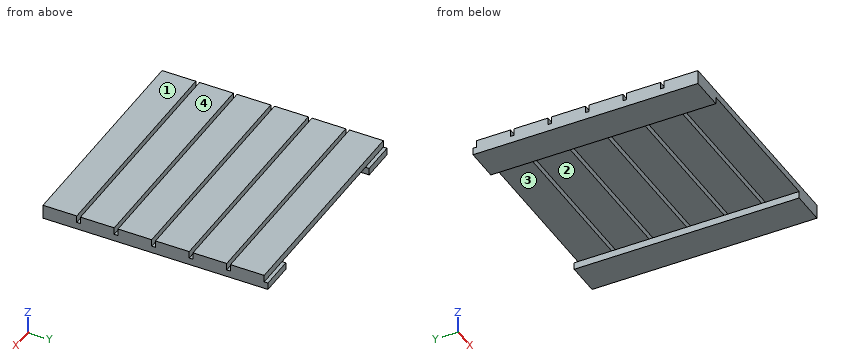
from build123d import *

# Parameters (mm, degrees)
BOX077_W     = 600
BOX077_H     = 90
BOX077_DEPTH = 19
BOX076_W     = 600
BOX076_H     = 90
BOX076_DEPTH = 19
BOX082_W     = 90
BOX082_H     = 600
BOX082_DEPTH = 19
BOX079_W     = 600
BOX079_H     = 90
BOX079_DEPTH = 19
BOX078_W     = 600
BOX078_H     = 90
BOX078_DEPTH = 19
BOX081_W     = 600
BOX081_H     = 90
BOX081_DEPTH = 19
BOX080_W     = 600
BOX080_H     = 90
BOX080_DEPTH = 19
BOX083_W     = 90
BOX083_H     = 600
BOX083_DEPTH = 19


with BuildPart() as cube049:
    # Box077 → Box077 (new body)
    with BuildSketch(Plane(origin=(0, 100, 0), x_dir=(1, 0, 0), z_dir=(0, 0, 1))):
        with Locations((300, 45)):
            Rectangle(BOX077_W, BOX077_H)
    extrude(amount=BOX077_DEPTH)


with BuildPart() as cube048:
    # Box076 → Box076 (new body)
    with BuildSketch(Plane.XY):
        with Locations((300, 45)):
            Rectangle(BOX076_W, BOX076_H)
    extrude(amount=BOX076_DEPTH)


with BuildPart() as cube054:
    # Box082 → Box082 (new body)
    with BuildSketch(Plane.XY.offset(-19)):
        with Locations((45, 300)):
            Rectangle(BOX082_W, BOX082_H)
    extrude(amount=BOX082_DEPTH)


with BuildPart() as cube051:
    # Box079 → Box079 (new body)
    with BuildSketch(Plane(origin=(0, 300, 0), x_dir=(1, 0, 0), z_dir=(0, 0, 1))):
        with Locations((300, 45)):
            Rectangle(BOX079_W, BOX079_H)
    extrude(amount=BOX079_DEPTH)


with BuildPart() as cube050:
    # Box078 → Box078 (new body)
    with BuildSketch(Plane(origin=(0, 200, 0), x_dir=(1, 0, 0), z_dir=(0, 0, 1))):
        with Locations((300, 45)):
            Rectangle(BOX078_W, BOX078_H)
    extrude(amount=BOX078_DEPTH)


with BuildPart() as cube053:
    # Box081 → Box081 (new body)
    with BuildSketch(Plane(origin=(0, 500, 0), x_dir=(1, 0, 0), z_dir=(0, 0, 1))):
        with Locations((300, 45)):
            Rectangle(BOX081_W, BOX081_H)
    extrude(amount=BOX081_DEPTH)


with BuildPart() as cube052:
    # Box080 → Box080 (new body)
    with BuildSketch(Plane(origin=(0, 400, 0), x_dir=(1, 0, 0), z_dir=(0, 0, 1))):
        with Locations((300, 45)):
            Rectangle(BOX080_W, BOX080_H)
    extrude(amount=BOX080_DEPTH)


with BuildPart() as obj1:
    # Box083 → Box083 (new body)
    with BuildSketch(Plane(origin=(510, 0, -19), x_dir=(1, 0, 0), z_dir=(0, 0, 1))):
        with Locations((45, 300)):
            Rectangle(BOX083_W, BOX083_H)
    extrude(amount=BOX083_DEPTH)

    # Fusion014: union Cube049, Cube048, Cube054, Cube051, Cube050, Cube053, Cube052
    add(cube049.part)
    add(cube048.part)
    add(cube054.part)
    add(cube051.part)
    add(cube050.part)
    add(cube053.part)
    add(cube052.part)


with BuildPart() as obj1_1:
    # Fusion014 placement: moved
    add(obj1.part.moved(Location((335, -115, 19))))


solid = obj1_1.part
Check sheet for the modelled part. Datum: model origin and axes. Units: mm. Face numbers are marked on the shaded views. A direction names the side the tool comes from. Round coordinates to 2 decimals unless told otherwise and drop trailing zeros. Order: outer loops, then holes, each group sorted by start corner. A loop starts at its lowest first (then second) coordinate and runs counter-clockwise, first axis right, second up.
Q1. Cross-section at B-B, the plane z = 30.5. Enter the section's corners in (x, y), plus the area to 3 significant figures.
Filled sheet:
outline: (335, -115) - (935, -115) - (935, -25) - (335, -25) - close; (335, -15) - (935, -15) - (935, 75) - (335, 75) - close; (335, 85) - (935, 85) - (935, 175) - (335, 175) - close; (335, 185) - (935, 185) - (935, 275) - (335, 275) - close; (335, 285) - (935, 285) - (935, 375) - (335, 375) - close; (335, 385) - (935, 385) - (935, 475) - (335, 475) - close
area: 324,000 mm2
Q2. Draft check along X on the marked faces 1 and 2. Enter one of: pulls with the +X half, pulls with the -X half, needs draft (parallel to the pull), parting line crosses it, or undercut.
Filled sheet:
face 1: needs draft
face 2: undercut
Q3. Depth check by flat-ended pin: P1, Ø3, axis at x = 360.5, y = 377.5, coming from the +Z side; P2, Ø15, axis at x = 657, z = 31.5, coming from the +Y side; P3, Ø8, axis at x = 390, y = 82.5, coming from the +Z side; P4, Ø10, axis at x = 438, y = 118, coming from the -Z side. Enter the tip coordinate at first touch or a pass-through.
Filled sheet:
P1: stops at z = 19
P2: stops at y = 475
P3: stops at z = 38
P4: stops at z = 19
Q4. Cross-section at C-C, the plane y = 60.5. Enter the section's corners in (x, z).
Filled sheet:
outline: (335, 0) - (425, 0) - (425, 19) - (845, 19) - (845, 0) - (935, 0) - (935, 38) - (335, 38) - close
Q5. Cross-section at A-A, the plane x = 819.5. Enter the section's corners in (y, z), plus the area to 3 significant figures.
Filled sheet:
outline: (-115, 19) - (-25, 19) - (-25, 38) - (-115, 38) - close; (-15, 19) - (75, 19) - (75, 38) - (-15, 38) - close; (85, 19) - (175, 19) - (175, 38) - (85, 38) - close; (185, 19) - (275, 19) - (275, 38) - (185, 38) - close; (285, 19) - (375, 19) - (375, 38) - (285, 38) - close; (385, 19) - (475, 19) - (475, 38) - (385, 38) - close
area: 10,300 mm2
Q6. Scan lines: L1, parallel to Y at x = 873.5, z = 34.5; L2, parallel to X at y = 198.5, z = 8; L3, parallel to Z at x = 816, y = 274.5. Record each from-to range of solid material in increasing order.
Filled sheet:
L1: y = -115 to -25, -15 to 75, 85 to 175, 185 to 275, 285 to 375, 385 to 475
L2: x = 335 to 425, 845 to 935
L3: z = 19 to 38
Q7. Set-up check for the marked faces 3 and 4: record each of +Z, -Z, +X, -X, +Y, -Y from which the full face is reachable in a straight line by a thin tool's end or side.
Filled sheet:
face 3: -Z, +Y, -Y
face 4: +Z, +X, -X, +Y, -Y
